Here's how the part is built. I have some questions about the finished solid (model axes, mm). Face numbers are marked on the shaded views. A direction names the side the tool comes from. Coordinates: 2 decimals unless noted, no trailing zeros. Order: outer loops, then holes, each group sorted by start corner. A loop starts at its lowest first (then second) coordinate and runs counter-clockwise, first axis right, second up. Notation, with made-up numbers: (67, 38) -> (91, 38) arc R31 cw to (91, 62) -> close; hole circle Ø3 at (4.25, 13.5). An arc over 180 degrees is marked (long way). One line per item, written item: value. Start each with the question number.
```python
from build123d import *

# Parameters (mm, degrees)
SKETCH_W  = 5.6
SKETCH_H  = 1.7
PAD_DEPTH = 8


with BuildPart() as part:
    # Sketch → Pad (new body)
    with BuildSketch(Plane.XZ):
        with BuildLine():
            Line((-22.25, -3), (-19.25, -3))
            Line((-19.25, -3), (-19.25, 0))
            Line((-19.25, 0), (-10.5, 0))
            Line((-10.5, 0), (-10.5, 2.5))
            ThreePointArc((-5.5, 2.5), (-8, 5), (-10.5, 2.5))
            Line((-5.5, 2.5), (-5.5, 0))
            Line((-5.5, 0), (-2.5, 0))
            Line((-2.5, 0), (-2.5, 2.5))
            ThreePointArc((2.5, 2.5), (0, 5), (-2.5, 2.5))
            Line((2.5, 2.5), (2.5, 0))
            Line((2.5, 0), (5.5, 0))
            Line((5.5, 0), (5.5, 2.5))
            ThreePointArc((10.5, 2.5), (8, 5), (5.5, 2.5))
            Line((10.5, 2.5), (10.5, 0))
            Line((10.5, 0), (19.25, 0))
            Line((19.25, 0), (19.25, -3))
            Line((19.25, -3), (22.25, -3))
            Line((22.25, -3), (22.25, 9))
            Line((22.25, 9), (14.25, 9))
            Line((14.25, 9), (14.25, 7))
            Line((14.25, 7), (-19.25, 7))
            Line((-19.25, 7), (-19.25, 10))
            Line((-19.25, 10), (-22.25, 10))
            Line((-22.25, 10), (-22.25, -3))
        make_face()
        with Locations((-16.45, 3.85)):
            Rectangle(SKETCH_W, SKETCH_H, mode=Mode.SUBTRACT)
        with Locations((16.45, 3.85)):
            Rectangle(SKETCH_W, SKETCH_H, mode=Mode.SUBTRACT)
    extrude(amount=PAD_DEPTH)


solid = part.part
```
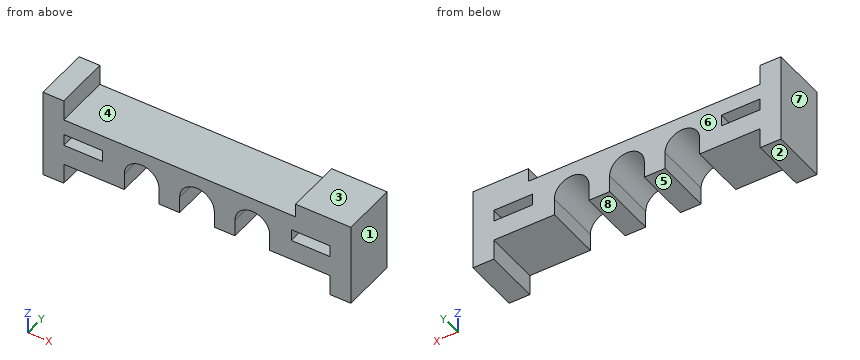
Q1. Imagine slicing it at A-A (x = -18). Write out the boundary of the cut face in (y, z).
Q2. If we mould it in two halves opening along X, with no side actions, what happens to the marked faces 6, 7 and 8? For each: +X half, -X half, draft (parallel to the pull), parting line (faces both ways), or undercut.
Q3. For P1, Ø1.7, axis at x = 17, y = -5, coming from the +Z side; P2, Ø1.5, axis at x = 9, y = -4.5, coming from the +Z side; P3, Ø1.5, axis at x = -4, y = -5.5, coming from the -Z side; P4, Ø6, axis at x = 9, z = 5.5, coming from the +Y side, each with a flat end and sliding along its axis, tell me the tip position at first contact or that it passes through.
Q4. Imagine slicing it at D-D (x = 11.5). Write out the boundary of the cut face in (y, z), plus the area to 3 significant figures.
Q5. I need wall thicknesses on line 1 (X direction, y = -4.5, z = 1.75); line 2 (Z direction, x = 15, y = -3.5); line 3 (X direction, y = -4, z = -0.75). Which ranges of each line are inside material? Lowest first, please.
Q6. Imagine slicing it at B-B (y = -4.5). Count the separate pieces of the cut face and the enclosed holes in it, plus the area to 3 significant figures.
Q7. Imagine slicing it at C-C (x = -8). Write out the boundary of the cut face in (y, z), plus the area to 3 significant figures.
Q8. For the marked faces 1, 2, 3, 4 and 5, which set-ups out of +Z, -Z, +X, -X, +Y, -Y let a thin tool reach every point of the face, with its end or its side?
Completed:
1. outline: (-8, 0) -> (0, 0) -> (0, 3) -> (-8, 3) -> close; (-8, 4.7) -> (0, 4.7) -> (0, 7) -> (-8, 7) -> close
2. face 6: draft
2. face 7: -X half
2. face 8: undercut
3. P1: stops at z = 9
3. P2: stops at z = 7
3. P3: stops at z = 0
3. P4: stops at y = 0
4. outline: (-8, 0) -> (0, 0) -> (0, 7) -> (-8, 7) -> close
4. area: 56.0 mm2
5. line 1: x = -22.25 to -10.5, -5.5 to -2.5, 2.5 to 5.5, 10.5 to 22.25
5. line 2: z = 0 to 3, 4.7 to 9
5. line 3: x = -22.25 to -19.25, 19.25 to 22.25
6. separate pieces: 1
6. enclosed holes: 2
6. area: 269 mm2
7. outline: (-8, 5) -> (0, 5) -> (0, 7) -> (-8, 7) -> close
7. area: 16.0 mm2
8. face 1: +Z, -Z, +X, +Y, -Y
8. face 2: -Z, +X, -X, +Y, -Y
8. face 3: +Z, +X, +Y, -Y
8. face 4: +Z, +Y, -Y
8. face 5: -Z, +Y, -Y
